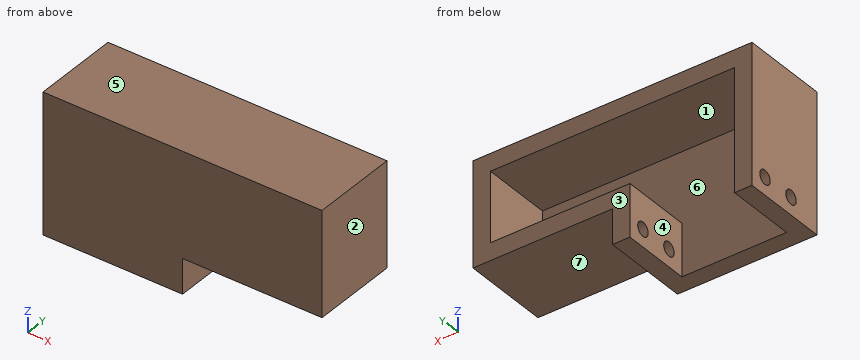
Autodesk Inventor part; units mm, degrees
ref_plane "XZ Plane" through (0, 0, 0) normal (0, 1, 0) x (-1, 0, 0)
ref_plane "XY Plane" through (0, 0, 0) normal (0, 0, 1) x (1, 0, 0)
sketch "Sketch1" plane through (0, 0, 0) normal (0, 0, 1) x (1, 0, 0)
  line L0 (-50.8, -15.875) -> (50.8, -15.875)
  line L1 (50.8, -15.875) -> (50.8, 15.875)
  line L2 (50.8, 15.875) -> (-50.8, 15.875)
  line L3 (-50.8, 15.875) -> (-50.8, -15.875)
  line L4 (-50.8, -15.875) -> (50.8, 15.875) construction
  line L5 (50.8, -15.875) -> (-50.8, 15.875) construction
  point P0 (0, 0)
  dimension "d0" = 101.6
  dimension "d1" = 31.75
extrude "Extrusion1" add sketch "Sketch1" along normal mid plane 38.1
sketch "Sketch3" plane through (-50.8, 15.875, 19.05) normal (0, 1, 0) x (1, 0, 0)
  line L0 (95.25, 6.35) -> (95.25, 31.75)
  line L1 (95.25, 31.75) -> (6.35, 31.75)
  line L2 (6.35, 31.75) -> (6.35, 6.35)
  line L3 (6.35, 6.35) -> (95.25, 6.35)
  line L4 (95.25, 6.35) -> (6.35, 31.75) construction
  line L5 (95.25, 31.75) -> (6.35, 6.35) construction
  line L6 (0, 38.1) -> (0, 0)
  line L7 (0, 38.1) -> (101.6, 38.1)
  point P0 (50.8, 19.05)
  dimension "d4" = 6.35
  dimension "d5" = 6.35
extrude "Extrusion2" cut sketch "Sketch3" against normal blind 25.4
sketch "Sketch8" plane through (-44.45, 15.875, -12.7) normal (0, 0, 1) x (1, 0, 0)
  line L0 (88.9, 0) -> (0, 0)
  line L1 (0, 0) -> (38.1, 0)
  line L2 (38.1, 0) -> (38.1, -25.4)
  line L3 (38.1, -25.4) -> (0, -25.4)
  line L4 (0, -25.4) -> (0, 0)
  point P0 (44.45, -15.875)
  dimension "d14" = 38.1
  dimension "d15" = 25.4
extrude "Extrusion5" cut sketch "Sketch8" against normal through all
sketch "Sketch9" plane through (0, 0, -19.05) normal (0, 0, -1) x (-1, 0, 0)
  line L0 (50.8, -15.875) -> (50.8, 15.875)
  line L1 (50.8, 15.875) -> (50.8, -15.875)
  line L2 (50.8, -15.875) -> (0, -15.875)
  line L3 (-50.8, -15.875) -> (50.8, -15.875)
  line L4 (0, -15.875) -> (0, 15.875)
  line L5 (-50.8, 15.875) -> (50.8, 15.875)
  line L6 (6.35, -9.525) -> (6.35, 15.875)
  line L7 (6.35, 15.875) -> (6.35, -9.525)
  line L8 (44.45, 15.875) -> (44.45, -9.525)
  line L9 (6.35, -9.525) -> (44.45, -9.525)
  line L10 (44.45, -9.525) -> (44.45, 15.875)
  line L11 (44.45, 15.875) -> (50.8, 15.875)
  point P0 (0, 0)
  dimension "d18" = 50.8
extrude "Extrusion6" add sketch "Sketch9" along normal blind 12.7 contours L2 L4 L5 L6 L9 L8 L0
sketch "Sketch10" plane through (0, -15.875, -19.05) normal (1, 0, 0) x (0, 0, -1)
  line L0 (12.7, 31.75) -> (-38.1, 31.75) construction
  line L1 (6.35, 31.75) -> (6.35, 0) construction
  line L2 (-38.1, 0) -> (12.7, 0) construction
  line L3 (12.7, 31.75) -> (12.7, 0) construction
  point P0 (-19.05, 15.875)
  point P1 (6.35, 25.4)
  point P2 (6.35, 12.7)
  dimension "d21" = 6.35
  dimension "d22" = 6.35
  dimension "d32" = 12.7
hole "Hole1" at (0, 9.525, -25.4) at (0, -3.175, -25.4) direction (-1, 0, 0) diameter 5.1054 end through all
properties part number "hookSupport" material "PBT Plastic"
Geometry check sheet. Reference: the model listing, model coordinates, mm. Face numbers are marked on the shaded views. A direction names the side the tool comes from. Coordinates: 2 decimals unless noted, no trailing zeros. Order: outer loops, then holes, each group sorted by start corner. A loop starts at its lowest first (then second) coordinate and runs counter-clockwise, first axis right, second up.
Q1. Sectioned sample at B-B on x = 12. Record the cut outline in (y, z) (3 decimals), and give its area (3 significant figures).
Reply:
outline: (-15.875, -19.05) - (15.875, -19.05) - (15.875, -12.7) - (-9.525, -12.7) - (-9.525, 12.7) - (15.875, 12.7) - (15.875, 19.05) - (-15.875, 19.05) - close
area: 565 mm2
Q2. Sectioned sample at D-D on y = -2. Record the cut outline in (x, z), and give its area (3 significant figures).
Reply:
outline: (-50.8, -31.75) - (-44.45, -31.75) - (-44.45, -27.67) - (-50.8, -27.67) - close; (-50.8, -23.13) - (-44.45, -23.13) - (-44.45, 12.7) - (44.45, 12.7) - (44.45, -12.7) - (-6.35, -12.7) - (-6.35, -23.13) - (0, -23.13) - (0, -19.05) - (50.8, -19.05) - (50.8, 19.05) - (-50.8, 19.05) - close; (-6.35, -31.75) - (0, -31.75) - (0, -27.67) - (-6.35, -27.67) - close
area: 1,470 mm2
Q3. Thickness scan on probe 1 along Y at (x, z) = (-47.75, -25.4) (3 decimals); probe 2 along Z at (x, y) = (4, 14.5); probe 3 along X at (y, z) = (5, 7.5). Record the ranges inside material, lowest first.
Reply:
probe 1: y = -15.875 to -5.728, -0.622 to 6.972, 12.078 to 15.875
probe 2: z = -19.05 to -12.7, 12.7 to 19.05
probe 3: x = -50.8 to -44.45, 44.45 to 50.8
Q4. Depth check by flat-ended pin: pin 1 Ø4 at (y, z) = (-1, -23.5) entering from +X; pin 2 Ø16 at (x, y) = (31, 6) entering from -Z. Enter the tip coordinate at first touch or a pass-through.
Reply:
pin 1: stops at x = 0
pin 2: stops at z = -19.05
Q5. Sectioned sample at C-C on z = -10.5. Record the cut outline in (x, y) (3 decimals), and give its area (3 significant figures).
Reply:
outline: (-50.8, -15.875) - (50.8, -15.875) - (50.8, 15.875) - (44.45, 15.875) - (44.45, -9.525) - (-44.45, -9.525) - (-44.45, 15.875) - (-50.8, 15.875) - close
area: 968 mm2
Q6. Draft check along X on the marked faces 1, 2 and 3. Enter one of: released by +X, released by -X, zero draft, split by the parting line, or undercut.
Reply:
face 1: undercut
face 2: released by +X
face 3: zero draft
Q7. Sectioned sample at A-A on z = -25.4. Record the cut outline in (x, y) (3 decimals).
Reply:
outline: (-50.8, -15.875) - (0, -15.875) - (0, -5.728) - (-6.35, -5.728) - (-6.35, -9.525) - (-44.45, -9.525) - (-44.45, -5.728) - (-50.8, -5.728) - close; (-50.8, -0.622) - (-44.45, -0.622) - (-44.45, 6.972) - (-50.8, 6.972) - close; (-50.8, 12.078) - (-44.45, 12.078) - (-44.45, 15.875) - (-50.8, 15.875) - close; (-6.35, -0.622) - (0, -0.622) - (0, 6.972) - (-6.35, 6.972) - close; (-6.35, 12.078) - (0, 12.078) - (0, 15.875) - (-6.35, 15.875) - close
Q8. Tool access check on the marked faces 4, 5, 6 and 7. Record the directions out of +Z, -Z, +X, -X, +Y, -Y that give a thin tool (end or side, any length) a straight path to the whole face; none if there is none.
Reply:
face 4: -Z, +Y
face 5: +Z, +X, -X, +Y, -Y
face 6: +Y
face 7: -Z, +X, +Y, -Y
